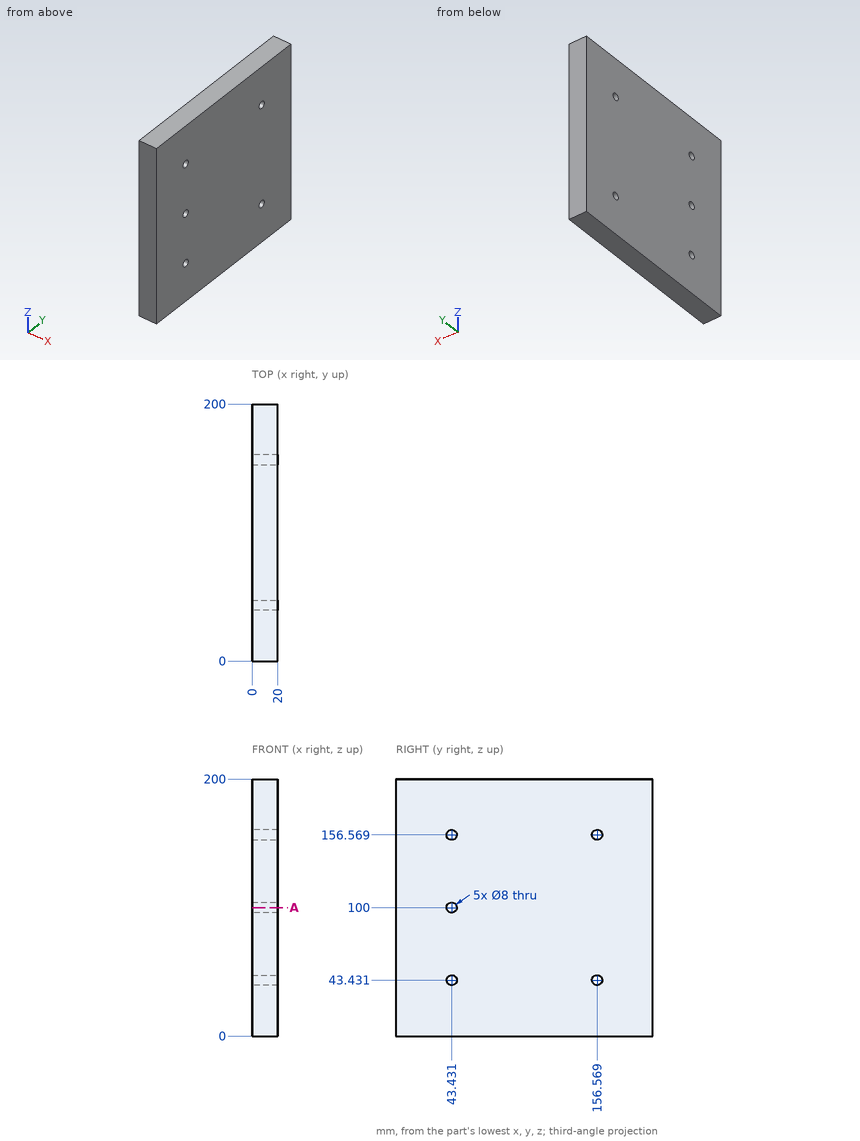
Source: three-view drawing plus pictorial views. Frame: mm from the lowest corner of the part. Round coordinates to 2 decimals unless told otherwise and drop trailing zeros. Loops run counter-clockwise (first coordinate to the right, second up) from the corner with the lowest first, then second, coordinate; pieces in that order, holes last.
Q1. Material intervals for L1, parallel to Y at x = 13.5, z = 158.5 (1 decimal); L2, parallel to Y at x = 16, z = 157.5; L3, parallel to Z at x = 13.75, y = 47 (1 decimal), sorted ascending.
Q2. Pin query (flat end, axial travel): P1, Ø1, axis at y = 68.5, z = 124.5, coming from the -X side; P2, Ø7, axis at y = 43.43, z = 43.43, coming from the +X side. Return the tip coordinate at first contact, or that it passes through.
Q3. Section A-A on z = 100. Return loops of the section in (x, y), plus the area to 3 significant figures.
Evaluation:
1. L1: y = 0 to 39.9, 46.9 to 153.1, 160.1 to 200
1. L2: y = 0 to 39.54, 47.32 to 152.68, 160.46 to 200
1. L3: z = 0 to 41.6, 45.2 to 98.2, 101.8 to 154.8, 158.4 to 200
2. P1: stops at x = 0
2. P2: passes through
3. outline: (0, 0) - (20, 0) - (20, 39.43) - (0, 39.43) - close; (0, 47.43) - (20, 47.43) - (20, 200) - (0, 200) - close
3. area: 3,840 mm2
